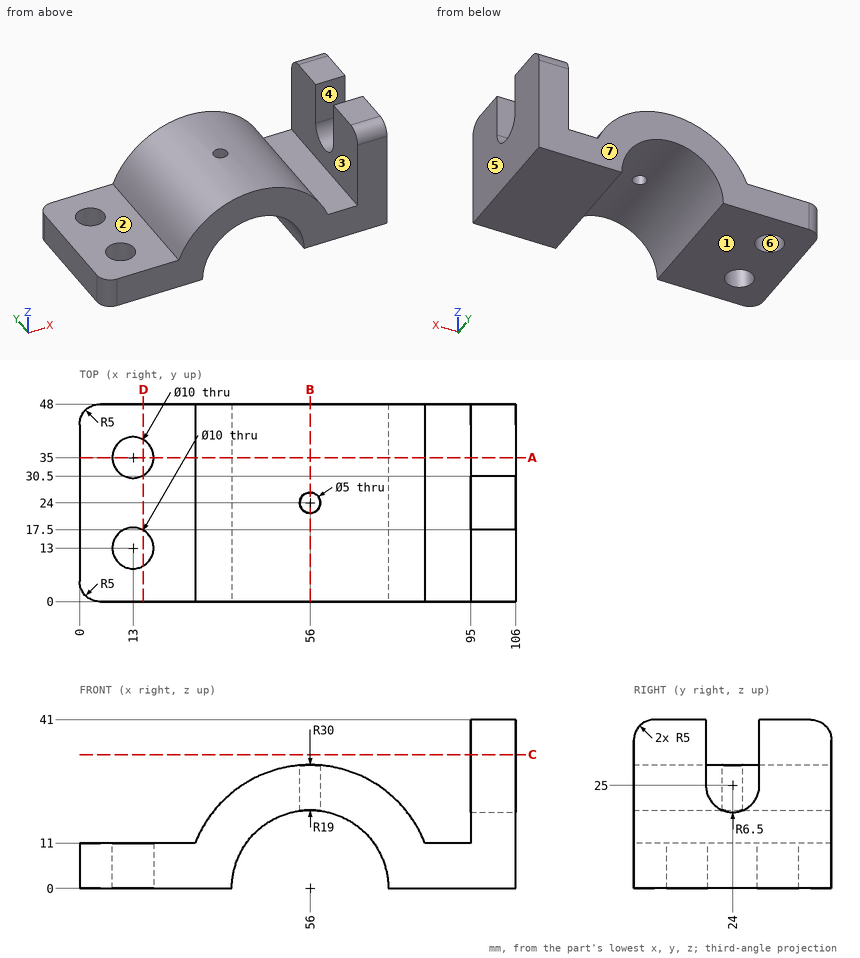
Could you check a few things on this drawing? It's one solid part, dimensions in mm from its lowest x, y, z. A direction names the side the tool comes from. Coordinates: 2 decimals unless noted, no trailing zeros. Order: outer loops, then holes, each group sorted by start corner. A loop starts at its lowest first (then second) coordinate and runs counter-clockwise, first axis right, second up.
1) Will these pins go through, and if not, where does the flat tip stop? pin 1 (6 mm diameter, centred on y = 33.5, z = 28, fed in from -X); pin 2 (9 mm diameter, centred on x = 13, y = 13, fed in from +Z); pin 3 (12 mm diameter, centred on x = 87.5, y = 26.5, fed in from +Z); pin 4 (1.5 mm diameter, centred on x = 56, y = 6, fed in from -Z).
2) Imagine slicing it at D-D on x = 15.5. List the corners of the cut face in (y, z) for me, and give its area (3 significant figures).
3) Imagine slicing it at A-A on y = 35. List the corners of the cut face in (x, z) for me, and give its area (3 significant figures).
4) Which directions (+Z, -Z, +X, -X, +Y, -Y) give clear straight access to the entire face, cutting with the end or side of a thin tool? Please do the marked faces 1, 2, 3 and 4.
5) We'd pull the mould along X, two halves only. Please class the marked faces 5, 6 and 7: +X half, -X half, draft (parallel to the pull), parting line (faces both ways), or undercut.
6) Imagine slicing it at B-B on x = 56. List the corners of the cut face in (y, z) for me, and give its area (3 significant figures).
7) Imagine slicing it at C-C on z = 32.5. List the corners of the cut face in (x, y) for me, and give its area (3 significant figures).
8) I need wall thicknesses on line 1 (Y direction, x = 13, z = 5.5); line 2 (X direction, y = 36, z = 5); line 3 (Z direction, x = 96.5, y = 2). Which ranges of each line are inside material? Lowest first, please.
Response values:
1. pin 1: stops at x = 39.42
1. pin 2: passes through
1. pin 3: stops at z = 15.8
1. pin 4: stops at z = 18.99
2. outline: (0, 0) - (8.67, 0) - (8.67, 11) - (0, 11) - close; (17.33, 0) - (30.67, 0) - (30.67, 11) - (17.33, 11) - close; (39.33, 0) - (48, 0) - (48, 11) - (39.33, 11) - close
2. area: 337 mm2
3. outline: (0, 0) - (8, 0) - (8, 11) - (0, 11) - close; (18, 0) - (37, 0) arc R19 cw to (75, 0) - (106, 0) - (106, 41) - (95, 41) - (95, 11) - (83.91, 11) arc R30 ccw to (28.09, 11) - (18, 11) - close
3. area: 1,590 mm2
4. face 1: -Z, +X, -X, +Y, -Y
4. face 2: +Z, -X, +Y, -Y
4. face 3: +Z, +Y, -Y
4. face 4: +Z, +X
5. face 5: +X half
5. face 6: undercut
5. face 7: draft
6. outline: (0, 19) - (21.5, 19) - (21.5, 30) - (0, 30) - close; (26.5, 19) - (48, 19) - (48, 30) - (26.5, 30) - close
6. area: 473 mm2
7. outline: (95, 0) - (106, 0) - (106, 17.5) - (95, 17.5) - close; (95, 30.5) - (106, 30.5) - (106, 48) - (95, 48) - close
7. area: 385 mm2
8. line 1: y = 0 to 8, 18 to 30, 40 to 48
8. line 2: x = 0 to 8.1, 17.9 to 37.67, 74.33 to 106
8. line 3: z = 0 to 40
